The drawing under review shows one solid part. Ordinate dimensions are in mm from its lowest x, y, z. Coordinates: 2 decimals unless noted, no trailing zeros. Loops run counter-clockwise (first coordinate to the right, second up) from the corner with the lowest first, then second, coordinate; pieces in that order, holes last. Notation, with made-up numbers: M 80,59.5 L 139,59.5 A27 cw 139,91.5 Z; hole C 70,23 d1. An arc over 180 degrees is marked long. Use one line per item in the form item = value.
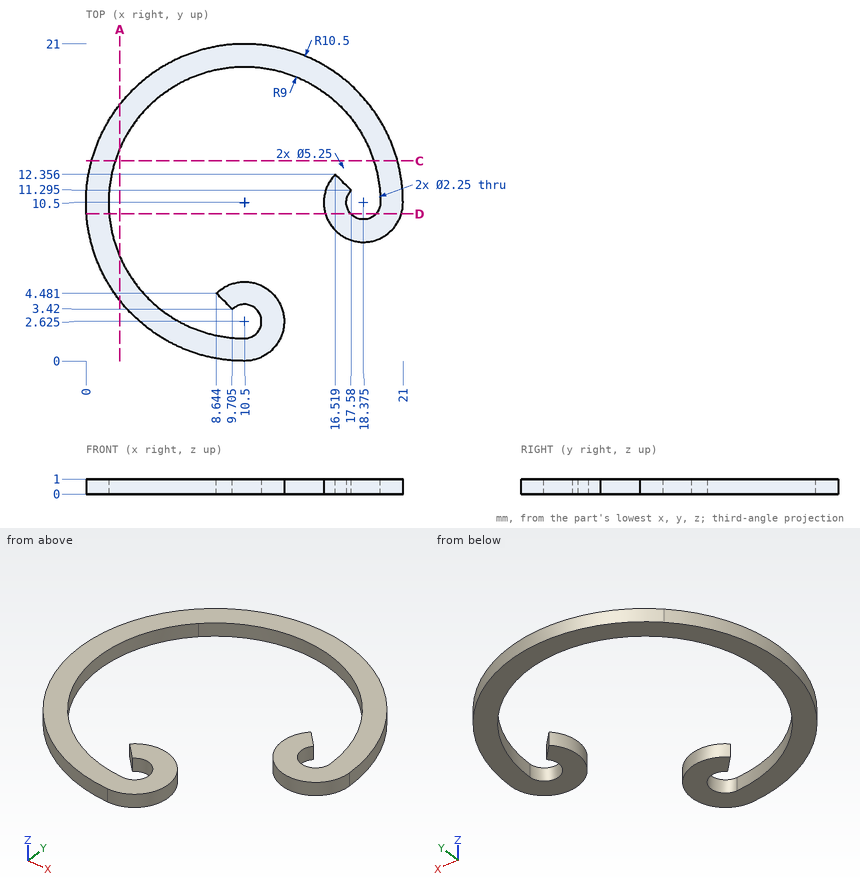
1. Consider section D-D on y = 9.75. Write out the cut boundary in (x, z).
Computed values:
outline = M 0.03,0 L 1.53,0 L 1.53,1 L 0.03,1 Z; M 15.86,0 L 17.54,0 L 17.54,1 L 15.86,1 Z; M 19.21,0 L 20.89,0 L 20.89,1 L 19.21,1 Z
2. Wall thickness on line 1 along Y through (x, z) = (10.5, 0.45); line 2 along Y through (x, z) = (4, 0.6) (1 decimal); line 3 along X through (y, z) = (8.25, 0.9) (1 decimal): over which ranges is each line inside the solid? List them lowest first. Write a range as from..to.
Computed values:
line_1 = 0..1.5, 3.75..5.25, 19.5..21
line_2 = 2.3..4.3, 16.7..18.7
line_3 = 0.2..1.8, 17..19.7
3. Consider section C-C on y = 13.25. Write out the cut boundary in (x, z).
Computed values:
outline = M 0.37,0 L 1.93,0 L 1.93,1 L 0.37,1 Z; M 19.07,0 L 20.63,0 L 20.63,1 L 19.07,1 Z
4. Consider section A-A on x = 2.25. Write out the cut boundary in (y, z) (1 decimal).
Computed values:
outline = M 4,0 L 6.9,0 L 6.9,1 L 4,1 Z; M 14.1,0 L 17,0 L 17,1 L 14.1,1 Z
5. For pin 1 Ø2 at (x, y) = (18.375, 10.5) entering from +Z; pin 2 Ø6 at (x, y) = (8, 17) entering from +Z, all flat-tipped, find the tip position at first contact; note any pin that passes through.
Computed values:
pin_1 = through
pin_2 = 1
